Input: part model. Units: mm. Frame: model coordinates. Round coordinates to 2 decimals unless told otherwise and drop trailing zeros. Loops run counter-clockwise (first coordinate to the right, second up) from the corner with the lowest first, then second, coordinate; pieces in that order, holes last. Notation, with made-up numbers: (31, 12.5) -> (78, 12.5) arc R9 ccw to (78, 23.5) -> close; hole circle Ø6 at (27.25, 66). An arc over 180 degrees is marked (long way). One line per question, with ' | ' between items. Start each with the question number.
Q1. Contact query for flat-ended pins moving along their axis: P1, Ø0.9, axis at x = -50, z = 0, coming from the +Y side; P2, Ø0.9, axis at y = -21.5, z = -0.5, coming from the -X side. Output: stop coordinate, or through.
Q2. Cut plane A-A on x = 49.5. Return loops of the section in (y, z).
Q3. Material intervals for L1, parallel to X at y = 1.5, z = 1.05; L2, parallel to Y at x = -49, z = -1.1, sorted ascending.
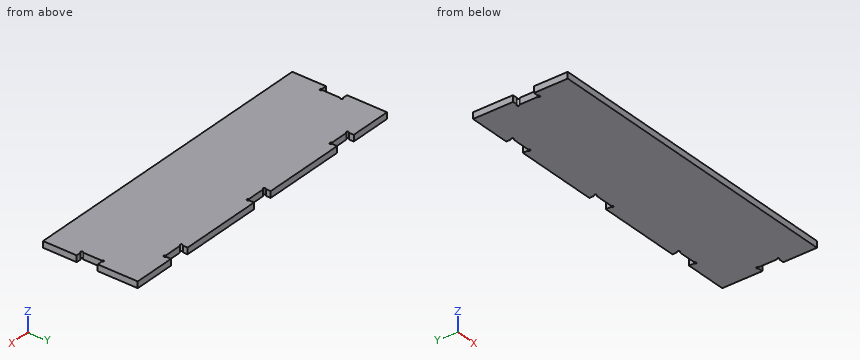
from build123d import *

# Parameters (mm, degrees)
BOSS_EXTRUDE1_DEPTH = 1.5
SKETCH2_R           = 0.5
CUT_EXTRUDE1_DEPTH  = 87.109465217
FILLET1_R           = 0.5


with BuildPart() as part:
    # Sketch1 → Boss-Extrude1 (new, symmetric)
    with BuildSketch(Plane.XY):
        Polygon((75, 3), (55, 3), (55, 0), (45, 0), (45, 3), (5, 3), (5, 0), (-5, 0), (-5, 3), (-45, 3), (-45, 0), (-55, 0), (-55, 3), (-75, 3), (-75, -16.1), (-72, -16.1), (-72, -26.1), (-75, -26.1), (-75, -42.2), (75, -42.2), (75, -26.1), (72, -26.1), (72, -16.1), (75, -16.1), align=None)
    extrude(amount=BOSS_EXTRUDE1_DEPTH, both=True)

    # Sketch2 → Cut-Extrude1 (cut, through all)
    with BuildSketch(Plane.XY.offset(1.5)):
        with Locations((-55, 0)):
            Circle(SKETCH2_R)
        with Locations((-45, 0)):
            Circle(SKETCH2_R)
        with Locations((-5, 0)):
            Circle(SKETCH2_R)
        with Locations((5, 0)):
            Circle(SKETCH2_R)
        with Locations((45, 0)):
            Circle(SKETCH2_R)
        with Locations((55, 0)):
            Circle(SKETCH2_R)
        with Locations((72, -16.1)):
            Circle(SKETCH2_R)
        with Locations((72, -26.1)):
            Circle(SKETCH2_R)
        with Locations((-72, -26.1)):
            Circle(SKETCH2_R)
        with Locations((-72, -16.1)):
            Circle(SKETCH2_R)
    extrude(amount=-CUT_EXTRUDE1_DEPTH, mode=Mode.SUBTRACT)

    # Fillet1
    fillet1_edges = [part.edges().sort_by_distance(p)[0] for p in [
        (-72, -25.6, 0),
        (-72.5, -26.1, 0),
        (72.5, -26.1, 0),
        (72, -25.6, 0),
        (72, -16.6, 0),
        (72.5, -16.1, 0),
        (55, 0.5, 0),
        (54.5, 0, 0),
        (45.5, 0, 0),
        (45, 0.5, 0),
        (5, 0.5, 0),
        (4.5, 0, 0),
        (-4.5, 0, 0),
        (-5, 0.5, 0),
        (-45, 0.5, 0),
        (-45.5, 0, 0),
        (-72.5, -16.1, 0),
        (-72, -16.6, 0),
        (-54.5, 0, 0),
        (-55, 0.5, 0),
    ]]
    fillet(fillet1_edges, radius=FILLET1_R)


solid = part.part
Results:
1) P1: y = 0 | P2: x = -72
2) outline: (-42.2, -1.5) -> (0, -1.5) -> (0, 1.5) -> (-42.2, 1.5) -> close
3) L1: -75 to -55, -45 to -5, 5 to 45, 55 to 75 | L2: -42.2 to 0
